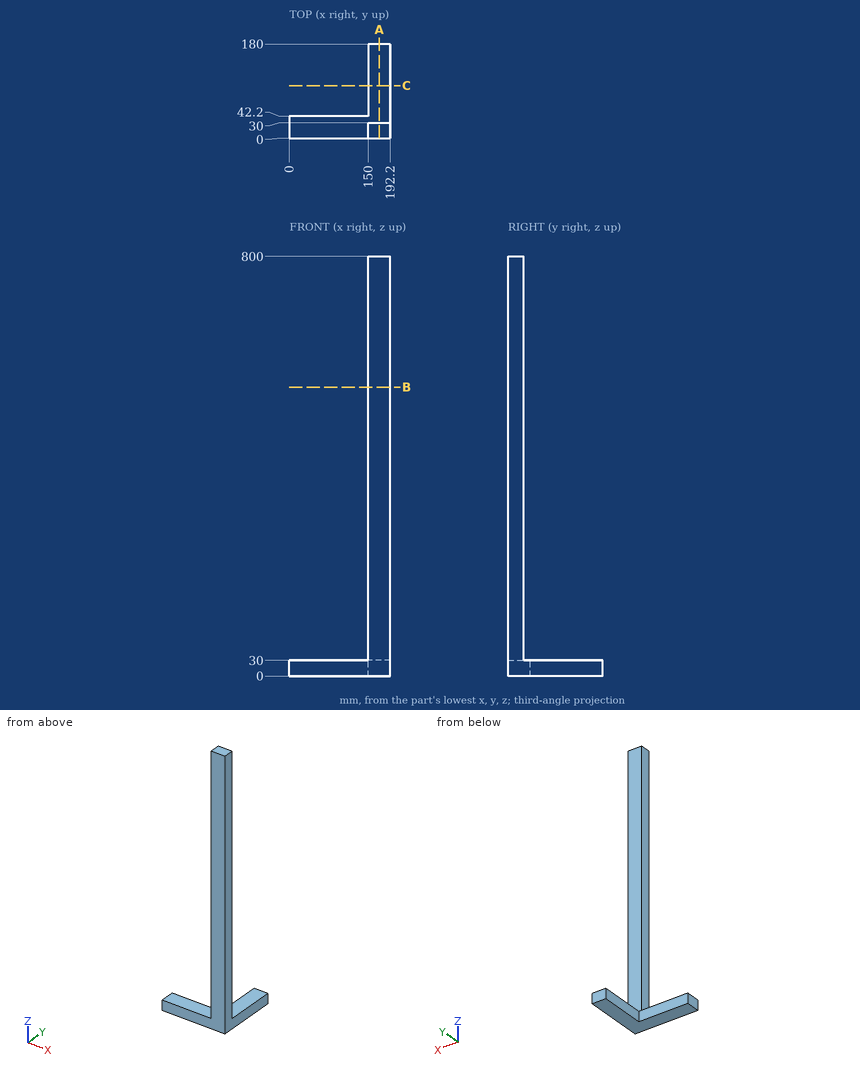
Drawing for the job (mm, zero at the part's lowest x, y, z). Round coordinates to 2 decimals unless told otherwise and drop trailing zeros. Order: outer loops, then holes, each group sorted by start corner. A loop starts at its lowest first (then second) coordinate and runs counter-clockwise, first axis right, second up.
Item 1: Probe line 1 along Z through (x, y) = (169.5, 121); line 2 along X through (y, z) = (24.5, 588). List the from-to ranges inside material, lowest first.
Item 2: Saw through at A-A on x = 171.5. Write the cut outline in (y, z).
Item 3: Pin check, flat tips, straight feed: pin 1 (24 mm diameter, centred on y = 120.5, z = 13.5, fed in from -X); pin 2 (12.5 mm diameter, centred on x = 172, z = 520.5, fed in from +Y); pin 3 (9 mm diameter, centred on x = 67.5, z = 21, fed in from +Y). Stop position of each tip, or through.
Item 4: Saw through at B-B on z = 551. Write the cut outline in (x, y).
Reported:
1. line 1: z = 0 to 30
1. line 2: x = 150 to 192.2
2. outline: (0, 0) - (180, 0) - (180, 30) - (30, 30) - (30, 800) - (0, 800) - close
3. pin 1: stops at x = 150
3. pin 2: stops at y = 30
3. pin 3: stops at y = 42.2
4. outline: (150, 0) - (192.2, 0) - (192.2, 30) - (150, 30) - close
